```python
from build123d import *

# Parameters (mm, degrees)
PAD_DEPTH            = 10
BODY_PLACEMENT_ANGLE = 90


with BuildPart() as part:
    # Sketch → Pad (new body)
    with BuildSketch(Plane.XY):
        Polygon((0, 0), (8, 0), (11.535534, 3.535534), (20, 3.535534), (20, 8.535534), (0, 8.535534), align=None)
    extrude(amount=PAD_DEPTH)


with BuildPart() as part_1:
    # Body placement: moved
    add(part.part.rotate(Axis((0, 0, 0), (1, 0, 0)), BODY_PLACEMENT_ANGLE))


solid = part_1.part
```
Geometry: final body of the model. Coordinates: model frame, mm. A direction names the side the tool comes from. Round coordinates to 2 decimals unless told otherwise and drop trailing zeros. Write each loop counter-clockwise with the first axis right and the second up, starting at its lowest first coordinate (ties: lowest second). Pieces come first, ordered by that corner, then holes.
Item 1: Section query A-A (y = -4.75). Return loops of the section in (x, z).
Item 2: Section query B-B (x = 10.25). Return loops of the section in (y, z), plus the area to 3 significant figures.
Item 3: Section query C-C (z = 2). Return loops of the section in (x, y), plus the area to 3 significant figures.
Item 4: Material intervals for L1, parallel to Z at x = 18.5, y = -8; L2, parallel to X at y = -1.75, z = 1; L3, parallel to X at y = -1.5, z = 2.25, sorted ascending.
Item 5: Pin query (flat end, axial travel): P1, Ø2.5, axis at x = 14, y = -2.5, coming from the -Z side; P2, Ø3, axis at x = 11.5, y = -5.5, coming from the -Z side. Return the tip coordinate at first contact, or that it passes through.
Item 6: Set-up query: faces 1 (the face through (16, -5, 3.536)), 2 (the face through (4, -5, 0)). Return all of +Z, -Z, +X, -X, +Y, -Y with unobstructed straight access to the full face (end or side cutting, diameter ignored); none if empty.
Completed:
1. outline: (0, 0) - (8, 0) - (11.54, 3.54) - (20, 3.54) - (20, 8.54) - (0, 8.54) - close
2. outline: (-10, 2.25) - (0, 2.25) - (0, 8.54) - (-10, 8.54) - close
2. area: 62.9 mm2
3. outline: (0, -10) - (10, -10) - (10, 0) - (0, 0) - close
3. area: 100 mm2
4. L1: z = 3.54 to 8.54
4. L2: x = 0 to 9
4. L3: x = 0 to 10.25
5. P1: stops at z = 3.54
5. P2: stops at z = 2
6. face 1: -Z, +X, +Y, -Y
6. face 2: -Z, +X, -X, +Y, -Y
